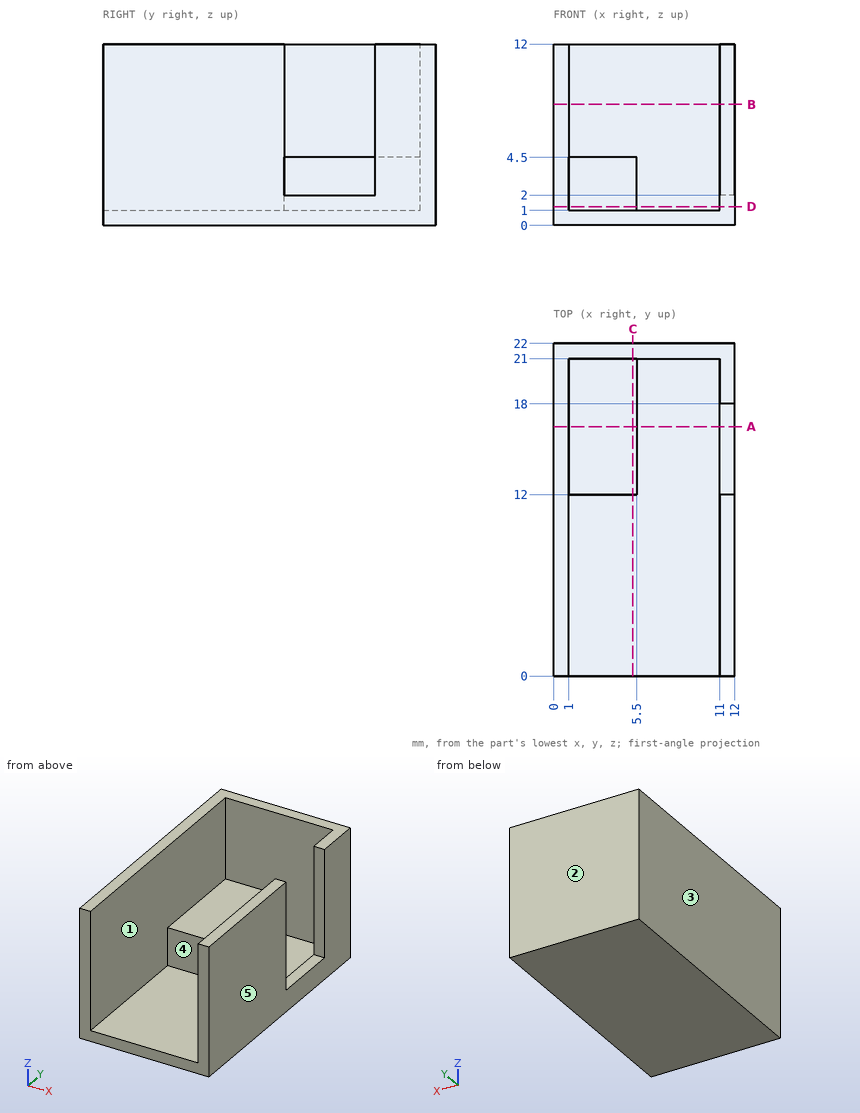
The drawing under review shows one solid part. Ordinate dimensions are in mm from its lowest x, y, z. A direction names the side the tool comes from. Give positions to 0.01 mm unless a question says otherwise; leave off trailing zeros. Write each loop counter-clockwise with the first axis right and the second up, starting at its lowest first coordinate (ties: lowest second). Pieces come first, ordered by that corner, then holes. Notation, with made-up numbers: M 28.5,-18 L 73.5,-18 A26 cw 73.5,19 Z; hole C 48.25,-2 d3. An arc over 180 degrees is marked long. Write each question's results on one line, items separated by ' | '. Start each with the question number.
1. For probe 1 along X at (y, z) = (20, 8.25); probe 2 along X at (y, z) = (14.5, 1.75); probe 3 along Y at (x, z) = (11.25, 10.75), list the stretches that pass through material, from the lowest coordinate up. Write a range as [from, to].
2. We need section A-A (y = 16.5). Write out the cut boundary in (x, z), and give its area (4 significant figures).
3. We need section C-C (x = 5.25). Write out the cut boundary in (y, z).
4. Insertion check: pin 1 Ø0.8 at (x, y) = (11.5, 14.5) entering from +Z; pin 2 Ø5 at (x, y) = (4.5, 17) entering from +Z; pin 3 Ø1 at (x, z) = (2.5, 3.5) entering from -Y. Each pin has a flat end and moves straight along its axis. Give the tip position at first contact, or say it passes through.
5. We need section B-B (z = 8). Write out the cut boundary in (x, y).
6. We need section D-D (z = 1.25). Write out the cut boundary in (x, y).
7. For the marked faces 4 and 5, list the 3-axis set-ups (+Z, -Z, +X, -X, +Y, -Y) from which the entire face can be reached by the end or side of a thin tool; tool diameter is ignored.
8. Mouldability with a two-part tool opening along X and no side actions: class the marked faces 1, 2 and 3 as released by +X, released by -X, zero draft, split by the parting line, or undercut.
Results found:
1) probe 1: x = [0, 1], [11, 12] | probe 2: x = [0, 5.5], [11, 12] | probe 3: y = [0, 12], [18, 22]
2) outline: M 0,0 L 12,0 L 12,2 L 11,2 L 11,1 L 5.5,1 L 5.5,4.5 L 1,4.5 L 1,12 L 0,12 Z | area: 39.75 mm^2
3) outline: M 0,0 L 22,0 L 22,12 L 21,12 L 21,4.5 L 12,4.5 L 12,1 L 0,1 Z
4) pin 1: stops at z = 2 | pin 2: stops at z = 4.5 | pin 3: stops at y = 12
5) outline: M 0,0 L 1,0 L 1,21 L 11,21 L 11,18 L 12,18 L 12,22 L 0,22 Z; M 11,0 L 12,0 L 12,12 L 11,12 Z
6) outline: M 0,0 L 1,0 L 1,12 L 5.5,12 L 5.5,21 L 11,21 L 11,0 L 12,0 L 12,22 L 0,22 Z
7) face 4: +Z, -Y | face 5: +Z, -Z, +X, +Y, -Y
8) face 1: undercut | face 2: zero draft | face 3: released by -X
